Autodesk Inventor part; units mm, degrees
ref_plane "YZ Plane" through (0, 0, 0) normal (1, 0, 0) x (0, 1, 0)
ref_plane "XZ Plane" through (0, 0, 0) normal (0, 1, 0) x (-1, 0, 0)
ref_plane "XY Plane" through (0, 0, 0) normal (0, 0, 1) x (1, 0, 0)
sketch "Sketch1" plane through (0, 0, 0) normal (0, 1, 0) x (-1, 0, 0)
  circle A0 centre (7, 0) radius 6.25
  circle A1 centre (0, 15.5) radius 1.6
  circle A2 centre (-13.4234, 7.75) radius 1.6
  circle A3 centre (-13.4234, -7.75) radius 1.6
  circle A4 centre (0, -15.5) radius 1.6
  circle A5 centre (13.4234, -7.75) radius 1.6
  circle A6 centre (13.4234, 7.75) radius 1.6
  circle A7 centre (0, 0) radius 27.5
  dimension "d0" = 7
  dimension "d1" = 12.5
  dimension "d2" = 3.2
  dimension "d3" = 15.5
  dimension "d6" = 360
  dimension "d8" = 55
extrude "Extrusion1" add sketch "Sketch1" along normal blind 6
sketch "Sketch2" plane through (0, 6, 0) normal (0, 1, 0) x (1, 0, 0)
  circle A0 centre (0, 0) radius 19
  circle A1 centre (0, 0) radius 27.5
  dimension "d11" = 38
extrude "Extrusion2" add sketch "Sketch2" along normal blind 12
properties part number "motor_holder_test"
Verification items for the finished model (mm, model axes). A direction names the side the tool comes from. Coordinates: 2 decimals unless noted, no trailing zeros. Order: outer loops, then holes, each group sorted by start corner. A loop starts at its lowest first (then second) coordinate and runs counter-clockwise, first axis right, second up.
1. Release check for a two-part mould opening along Z. For faces 3 (the face through (6, 18, -19)), 4 (the face through (1.81, 8.87, 27.44)), 5 (the face through (0, 6, 0)) record: +Z half, -Z half, draft (parallel to the pull), parting line (faces both ways), or undercut.
Results found:
face 3: draft
face 4: parting line
face 5: undercut
2. Sectioned sample at C-C, the plane y = 15.75. Record the cut outline in (x, z).
Results found:
outline: circle Ø55 at (0, 0); hole circle Ø38 at (0, 0)
3. Go/stop test with flat-tipped pins: pin 1 Ø3.5 at (x, z) = (-13.42, 7.75) entering from +Y; pin 2 Ø5 at (x, z) = (13.42, 7.75) entering from -Y; pin 3 Ø6 at (x, y) = (0.5, 15.5) entering from +Z; pin 4 Ø3 at (x, y) = (10, 14) entering from -Z. Record where each tip stops, or that it passes through.
Results found:
pin 1: stops at y = 6
pin 2: stops at y = 0
pin 3: stops at z = 27.5
pin 4: stops at z = -26.15
4. Set-up check for faces 1 (the face through (11.945, 2.958, 8.363)), 2 (the face through (8.767, 11.916, -16.856)): record each of +Z, -Z, +X, -X, +Y, -Y from which the full face is reachable in a straight line by a thin tool's end or side.
Results found:
face 1: +Y, -Y
face 2: +Y
5. Sectioned sample at B-B, the plane z = -7. Record the cut outline in (x, y).
Results found:
outline: (-26.59, 0) - (-14.84, 0) - (-14.84, 6) - (-17.66, 6) - (-17.66, 18) - (-26.59, 18) - close; (-12.01, 0) - (12.01, 0) - (12.01, 6) - (-12.01, 6) - close; (14.84, 0) - (26.59, 0) - (26.59, 18) - (17.66, 18) - (17.66, 6) - (14.84, 6) - close
6. Scan lines: line 1 (Z direction, x = 0, y = 4.4); line 2 (X direction, y = 8.5, z = 0); line 3 (Y direction, x = 14, z = -12.5). Record each from-to range of solid material in increasing order.
Results found:
line 1: z = -27.5 to -17.1, -13.9 to 13.9, 17.1 to 27.5
line 2: x = -27.5 to -19, 19 to 27.5
line 3: y = 0 to 6
